from build123d import *

# Parameters (mm, degrees)
F0_R        = 21.25
F0_R_2      = 18.75
F1_DEPTH    = 20
F3_R        = 21.25
F3_R_2      = 18
F4_DEPTH    = 25
F4_FACE_R   = 21.25
F4_FACE_R_2 = 18
F5_DEPTH    = 8
F7_W        = 6
F7_H        = 2.5
F8_ANGLE    = 20
F9_W        = 8
F9_H        = 2.5
F10_ANGLE   = 190


with BuildPart() as f1:
    # F0 (on Front) → F1 (new body)
    with BuildSketch(Plane.XZ):
        Circle(F0_R)
        Circle(F0_R_2, mode=Mode.SUBTRACT)
    extrude(amount=F1_DEPTH)


with BuildPart() as f4:
    # F3 (on offset) → F4 (new body)
    with BuildSketch(Plane.XZ.offset(28)):
        Circle(F3_R)
        Circle(F3_R_2, mode=Mode.SUBTRACT)
    extrude(amount=F4_DEPTH)


with BuildPart() as f5:
    # F4_face (on face) → F5 (new body, through all)
    with BuildSketch(Plane(origin=(0, -28, 0), x_dir=(1, 0, 0), z_dir=(0, 1, 0))):
        Circle(F4_FACE_R)
        Circle(F4_FACE_R_2, mode=Mode.SUBTRACT)
    extrude(amount=F5_DEPTH)


with BuildPart() as f1_1:
    add(f1.part)

    # F6: union F4, F5
    add(f4.part)
    add(f5.part)

    # F7 (on Right) → F8 (revolve)
    with BuildSketch(Plane.YZ):
        with Locations((3, 20)):
            Rectangle(F7_W, F7_H)
    revolve(axis=Axis((0, 6.62554, 0), (0, 1, 0)), revolution_arc=F8_ANGLE)

    # F9 (on face) → F10 (revolve)
    with BuildSketch(Plane(origin=(0, 0, 0), x_dir=(0, -1, 0), z_dir=(-1, 0, 0))):
        with Locations((-10, 20)):
            Rectangle(F9_W, F9_H)
    revolve(axis=Axis((0, 8.909439, 0), (0, 1, 0)), revolution_arc=F10_ANGLE)


solid = f1_1.part
The listing builds one solid part. Answer for the finished solid, in the listing's coordinates (mm). A direction names the side the tool comes from. Coordinates: 2 decimals unless noted, no trailing zeros. Order: outer loops, then holes, each group sorted by start corner. A loop starts at its lowest first (then second) coordinate and runs counter-clockwise, first axis right, second up. Notation, with made-up numbers: (-31, -27.5) -> (18, -27.5) arc R26 cw to (18, 11.5) -> close; hole circle Ø11 at (-28, -28.75). An arc over 180 degrees is marked (long way). Answer in a Markdown table with one row per item. Add a question column.
Item 1: Which of the six approach directions +Z, -Z, +X, -X, +Y, -Y give full straight-line access (tool end or side, diameter ignored) to faces 4 (the face through (-16, -53, 10)), 5 (the face through (-3.476, 10.056, -19.713)), 6 (the face through (6.846, 2.958, 18.81))?
Item 2: Find section A-A (z = -9.5). Write down the section's boundary in (x, y).
Item 3: Find section D-D (y = -36). Write down the section's boundary in (x, z).
Item 4: Find the intervals of material crossed by L1, parallel to X at y = -13, z = 0; L2, parallel to X at y = -45, z = 0.5; L3, parallel to Y at x = 11.5, z = -16, in increasing order. Write a range as from..to.
Item 5: Determine the mould class of faces 1 (the face through (19, 14, -1)), 2 (the face through (-17, -20, -7)), 3 (the face through (0, 7, 20)) for opening direction X: +X half, -X half, draft (parallel to the pull), parting line (faces both ways), or undercut.
Item 6: Find section B-B (x = 9.5). Write down the section's boundary in (y, z), then the cut area to 3 significant figures.
Item 7: Find section C-C (z = 0). Write down the section's boundary in (x, y).
Item 8: Each of these flat-tipped pins is pushed along its axis until it touches: P1, Ø10, axis at x = -6, z = -11, coming from the +Y side; P2, Ø12, axis at x = 13.5, y = 3.5, coming from the -Z side; P3, Ø10, axis at x = 11, y = -35, coming from the -Z side; P4, Ø4, axis at x = 2.5, y = -2, coming from the -Z side. Where does it stop, or does it pass through?
Result set:
| question | item | result |
|---|---|---|
| 1 | face 4 | +Z, -Z, +X, -X, -Y |
| 1 | face 5 | +Z, -X, +Y |
| 1 | face 6 | -Z, +X |
| 2 | outline | (-19.01, -53) -> (-15.29, -53) -> (-15.29, -20) -> (-16.17, -20) -> (-16.17, 0) -> (-19.01, 0) -> close; (15.29, -53) -> (19.01, -53) -> (19.01, 0) -> (16.17, 0) -> (16.17, -20) -> (15.29, -20) -> close; (16.17, 6) -> (19.01, 6) -> (19.01, 14) -> (16.17, 14) -> close |
| 3 | outline | circle Ø42.5 at (0, 0); hole circle Ø36 at (0, 0) |
| 4 | L1 | x = -21.25..-18.75, 18.75..21.25 |
| 4 | L2 | x = -21.24..-17.99, 17.99..21.24 |
| 4 | L3 | y = -53..0, 6..14 |
| 5 | face 1 | draft |
| 5 | face 2 | undercut |
| 5 | face 3 | -X half |
| 6 | outline | (-53, -19.01) -> (0, -19.01) -> (0, -16.17) -> (-20, -16.17) -> (-20, -15.29) -> (-53, -15.29) -> close; (-53, 15.29) -> (-20, 15.29) -> (-20, 16.17) -> (0, 16.17) -> (0, 19.01) -> (-53, 19.01) -> close; (6, -19.01) -> (14, -19.01) -> (14, -16.17) -> (6, -16.17) -> close; (6, 16.17) -> (14, 16.17) -> (14, 19.01) -> (6, 19.01) -> close |
| 6 | area | 405 mm² |
| 7 | outline | (-21.25, -53) -> (-18, -53) -> (-18, -20) -> (-18.75, -20) -> (-18.75, 0) -> (-21.25, 0) -> close; (18, -53) -> (21.25, -53) -> (21.25, 0) -> (18.75, 0) -> (18.75, -20) -> (18, -20) -> close; (18.75, 6) -> (21.25, 6) -> (21.25, 14) -> (18.75, 14) -> close |
| 8 | P1 | passes through |
| 8 | P2 | stops at z = -19.67 |
| 8 | P3 | stops at z = -20.39 |
| 8 | P4 | stops at z = -21.24 |
